Autodesk Inventor part; units mm, degrees
ref_plane "Deaktiviert_NICHT_mehrverwenden_Zyl__Schraube_DIN_EN_ISO_4762_XY" through (0, 0, 0) normal (0, 1, 0) x (1, 0, 0)
ref_plane "Deaktiviert_NICHT_mehrverwenden_Zyl__Schraube_DIN_EN_ISO_4762_YZ" through (0, 0, 0) normal (1, 0, 0) x (0, 0, -1)
ref_plane "Deaktiviert_NICHT_mehrverwenden_Zyl__Schraube_DIN_EN_ISO_4762_ZX" through (0, 0, 0) normal (0, 0, -1) x (0, 1, 0)
sketch "Skizze_1" plane through (0, 0, 0) normal (0, 0, 1) x (1, 0, 0)
  line L0 (0, -30) -> (0, 0)
  line L1 (0, 0) -> (4, 0)
  line L2 (4, 0) -> (4, -29.233)
  line L3 (4, -29.233) -> (3.233, -30)
  line L4 (3.233, -30) -> (0, -30)
  line L5 (0, -30) -> (0, 0)
revolve "Revolution1" add sketch "Skizze_1" angle 360 about axis through (0, -30, 0) along (0, -1, 0)
thread "Thread1"
sketch "Skizze_2" plane through (0, 0, 0) normal (0, 0, 1) x (1, 0, 0)
  line L0 (0, 0) -> (0, 5)
  line L1 (0, 5) -> (6, 5)
  arc A0 (6.5, 4.5) -> (6, 5) centre (6, 4.5) ccw
  line L2 (6.5, 4.5) -> (6.5, 0)
  line L3 (6.5, 0) -> (0, 0)
  line L4 (0, 0) -> (0, 5)
revolve "Revolution2" add sketch "Skizze_2" angle 360 about axis through (0, 0, 0) along (0, -1, 0)
sketch "Skizze_3" plane through (0, 5, 0) normal (0, 1, 0) x (1, 0, 0)
  line L0 (-2.5, -1.4434) -> (0, -2.8868)
  line L1 (0, -2.8868) -> (2.5, -1.4434)
  line L2 (2.5, -1.4434) -> (2.5, 1.4434)
  line L3 (2.5, 1.4434) -> (0, 2.8868)
  line L4 (0, 2.8868) -> (-2.5, 1.4434)
  line L5 (-2.5, 1.4434) -> (-2.5, -1.4434)
extrude "Extrusion1" cut sketch "Skizze_3" against normal blind 5
ref_plane "EP_XY" through (0, 0, 0) normal (0, 1, 0) x (1, 0, 0)
ref_plane "EP_YZ" through (0, 0, 0) normal (1, 0, 0) x (0, 0, -1)
ref_plane "EP_ZX" through (0, 0, 0) normal (0, 0, -1) x (0, 1, 0)
ref_plane "EP_Schraube_XY" through (0, 0, 0) normal (0, 1, 0) x (1, 0, 0)
ref_plane "EP_Schraube_YZ" through (0, 0, 0) normal (1, 0, 0) x (0, 0, -1)
ref_plane "EP_Schraube_ZX" through (0, 0, 0) normal (0, 0, -1) x (0, 1, 0)
properties part number "Zyl.Schr-M8x30_Stahl_X094960"
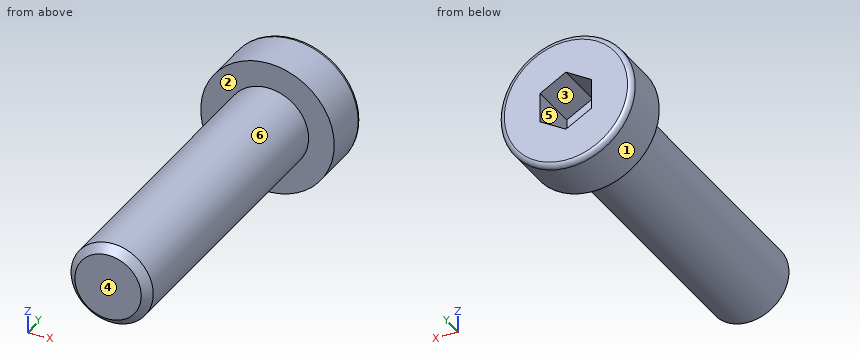
Design review of the part built by this model. Coordinates are the model's own, in mm. Face numbers are marked on the shaded views. A direction names the side the tool comes from. Round coordinates to 2 decimals unless told otherwise and drop trailing zeros. Write each loop counter-clockwise with the first axis right and the second up, starting at its lowest first coordinate (ties: lowest second). Pieces come first, ordered by that corner, then holes.
Item 1: For pin 1 Ø1 at (y, z) = (-22.5, 2.5) entering from -X; pin 2 Ø2 at (x, y) = (-3.5, -19.5) entering from -Z; pin 3 Ø6 at (y, z) = (-12.5, -0.5) entering from +X, all flat-tipped, find the tip position at first contact; note any pin that passes through.
Item 2: For the marked faces 1 and 2, list the 3-axis set-ups (+Z, -Z, +X, -X, +Y, -Y) from which the entire face can be reached by the end or side of a thin tool; tool diameter is ignored.
Item 3: Consider section B-B on y = -19. Give the boundary of the cut face in (x, z).
Item 4: Wall thickness on L1, parallel to Y at x = -3.25, z = -4.5; L2, parallel to Y at x = -0.25, z = -0.25; L3, parallel to Z at x = 3.25, y = -11.5: over which ranges is each line inside the solid? List them lowest first.
Item 5: Draft analysis for pull direction X (two halves, no side actions). For the marked faces 3, 4, 5 and 6, state which applies: released by +X, released by -X, zero draft, split by the parting line, or undercut.
Item 6: Consider section A-A on z = 0. Give the boundary of the cut face in (x, y).
Check values:
1. pin 1: stops at x = -3.46
1. pin 2: stops at z = -3.12
1. pin 3: stops at x = 4
2. face 1: +Y, -Y
2. face 2: -Y
3. outline: circle Ø8 at (0, 0)
4. L1: y = 0 to 5
4. L2: y = -30 to 0
4. L3: z = -2.33 to 2.33
5. face 3: undercut
5. face 4: zero draft
5. face 5: undercut
5. face 6: split by the parting line
6. outline: (-6.5, 0) - (-4, 0) - (-4, -29.23) - (-3.23, -30) - (3.23, -30) - (4, -29.23) - (4, 0) - (6.5, 0) - (6.5, 4.5) arc R0.5 ccw to (6, 5) - (2.5, 5) - (2.5, 0) - (-2.5, 0) - (-2.5, 5) - (-6, 5) arc R0.5 ccw to (-6.5, 4.5) - close
